```python
from build123d import *

# Parameters (mm, degrees)
SKETCH1_W                   = 26.12
SKETCH1_H                   = 24
SKETCH1_R                   = 1.25
BOSS_EXTRUDE1_DEPTH         = 2
SKETCH4_W                   = 26.12
SKETCH4_H                   = 2
BOSS_EXTRUDE4_DEPTH         = 20
FILLET2_R                   = 2.54
FILLET3_R                   = 1
FILLET4_R                   = 1
FILLET5_R                   = 1
BOSS_EXTRUDE5_DEPTH         = 2
BOSS_EXTRUDE6_DEPTH         = 1
FILLET10_R                  = 1
SKETCH15_R                  = 3.5
BOSS_EXTRUDE7_DEPTH         = 8
M3_5X0_6_TAPPED_HOLE1_D     = 2.9
M3_5X0_6_TAPPED_HOLE1_DEPTH = 10
M3_5X0_6_TAPPED_HOLE1_TIP   = 0.871247898
SKETCH19_R                  = 3.500559702
SKETCH19_R_2                = 1.27
BOSS_EXTRUDE8_DEPTH         = 3
CUT_EXTRUDE1_DEPTH          = 3
FILLET11_R                  = 2.54
SKETCH21_R                  = 1.75
CUT_EXTRUDE2_DEPTH          = 3


with BuildPart() as part:
    # Sketch1 → Boss-Extrude1 (new body)
    with BuildSketch(Plane.XY):
        with Locations((-15.65045068, 0.61225)):
            Rectangle(SKETCH1_W, SKETCH1_H)
        with Locations((-7.12045068, -2.85775)):
            Circle(SKETCH1_R, mode=Mode.SUBTRACT)
        with Locations((-24.18045068, 10.09225)):
            Circle(SKETCH1_R, mode=Mode.SUBTRACT)
    extrude(amount=BOSS_EXTRUDE1_DEPTH)

    # Sketch4 → Boss-Extrude4 (add)
    with BuildSketch(Plane(origin=(0, 0, 0), x_dir=(-1, 0, 0), z_dir=(0, 0, -1))):
        with Locations((15.65045068, -10.38775)):
            Rectangle(SKETCH4_W, SKETCH4_H)
    extrude(amount=BOSS_EXTRUDE4_DEPTH)

    # Fillet2
    fillet2_edges = [part.edges().sort_by_distance(p)[0] for p in [
        (-28.71045068, 12.61225, 1),
    ]]
    fillet(fillet2_edges, radius=FILLET2_R)

    # Fillet3
    fillet3_edges = [part.edges().sort_by_distance(p)[0] for p in [
        (-2.59045068, 12.61225, 1),
    ]]
    fillet(fillet3_edges, radius=FILLET3_R)

    # Fillet4
    fillet4_edges = [part.edges().sort_by_distance(p)[0] for p in [
        (-28.71045068, -10.38775, -20),
        (-2.59045068, -10.38775, -20),
    ]]
    fillet(fillet4_edges, radius=FILLET4_R)

    # Fillet5
    fillet5_edges = [part.edges().sort_by_distance(p)[0] for p in [
        (-15.65045068, -9.38775, 0),
    ]]
    fillet(fillet5_edges, radius=FILLET5_R)

    # Sketch7 → Boss-Extrude5 (add)
    with BuildSketch(Plane.XY.offset(2)):
        with BuildLine():
            Line((-26.610166349, 12.61225), (-21.750735012, 12.61225))
            ThreePointArc((-21.750735012, 12.61225), (-24.18045068, 13.592809702), (-26.610166349, 12.61225))
        make_face()
    extrude(amount=-BOSS_EXTRUDE5_DEPTH)

    # Sketch14 → Boss-Extrude6 (add, symmetric)
    with BuildSketch(Plane.ZY.offset(15.65045068)):
        Polygon((0, 11.61225), (-19, -9.38775), (0, -9.38775), (0, 11.544281389), align=None)
    extrude(amount=BOSS_EXTRUDE6_DEPTH, both=True)

    # Fillet10
    fillet10_edges = [part.edges().sort_by_distance(p)[0] for p in [
        (-14.65045068, -9.094856781, -0.292893219),
        (-16.65045068, -9.094856781, -0.292893219),
        (-14.65045068, 1.61225, 0),
        (-16.65045068, 1.61225, 0),
        (-16.65045068, -9.38775, -10),
        (-14.65045068, -9.38775, -10),
    ]]
    fillet(fillet10_edges, radius=FILLET10_R)

    # Sketch15 → Boss-Extrude7 (add)
    with BuildSketch(Plane.XZ.offset(11.38775)):
        with Locations((-15.65045068, -9)):
            Circle(SKETCH15_R)
    extrude(amount=-BOSS_EXTRUDE7_DEPTH)

    # M3.5x0.6 Tapped Hole1
    with Locations(Plane(origin=(0, -11.38775, 0), x_dir=(-1, 0, 0), z_dir=(0, -1, 0))):
        with Locations((15.65045068, 9)):
            Hole(M3_5X0_6_TAPPED_HOLE1_D / 2, depth=M3_5X0_6_TAPPED_HOLE1_DEPTH)
            with Locations((0, 0, -(M3_5X0_6_TAPPED_HOLE1_DEPTH + M3_5X0_6_TAPPED_HOLE1_TIP / 2))):  # 118° drill point
                Cone(0, M3_5X0_6_TAPPED_HOLE1_D / 2, M3_5X0_6_TAPPED_HOLE1_TIP, mode=Mode.SUBTRACT)

    # Sketch19 → Boss-Extrude8 (add)
    with BuildSketch(Plane(origin=(0, 0, 0), x_dir=(-1, 0, 0), z_dir=(0, 0, -1))):
        with Locations((7.12045068, -2.85775)):
            Circle(SKETCH19_R)
        with Locations((7.12045068, -2.85775)):
            Circle(SKETCH19_R_2, mode=Mode.SUBTRACT)
        with Locations((24.18045068, 10.09225)):
            Circle(SKETCH19_R)
        with Locations((24.18045068, 10.09225)):
            Circle(SKETCH19_R_2, mode=Mode.SUBTRACT)
    extrude(amount=BOSS_EXTRUDE8_DEPTH)

    # Sketch20 → Cut-Extrude1 (cut, through all)
    with BuildSketch(Plane(origin=(0, 0, 0), x_dir=(-1, 0, 0), z_dir=(0, 0, -1))):
        with BuildLine():
            Line((21.027116218, 11.61225), (2.59045068, 11.61225))
            Line((2.59045068, 11.61225), (2.59045068, 12.61225))
            Line((2.59045068, 12.61225), (21.750735012, 12.61225))
            ThreePointArc((21.750735012, 12.61225), (21.344500718, 12.144396691), (21.027116218, 11.61225))
        make_face()
    extrude(amount=-CUT_EXTRUDE1_DEPTH, mode=Mode.SUBTRACT)

    # Fillet11
    fillet11_edges = [part.edges().sort_by_distance(p)[0] for p in [
        (-2.59045068, 11.61225, 1),
    ]]
    fillet(fillet11_edges, radius=FILLET11_R)

    # Sketch21 → Cut-Extrude2 (cut, through all)
    with BuildSketch(Plane(origin=(0, -9.38775, 0), x_dir=(1, 0, 0), z_dir=(0, 1, 0))):
        with Locations((-23.63045068, 14.92)):
            Circle(SKETCH21_R)
        with Locations((-7.67045068, 14.92)):
            Circle(SKETCH21_R)
    extrude(amount=-CUT_EXTRUDE2_DEPTH, mode=Mode.SUBTRACT)


solid = part.part
```
Work out the finished part from the listing and answer in its coordinate system (mm). A direction names the side the tool comes from. Give positions to 0.01 mm unless a question says otherwise; leave off trailing zeros. Loops run counter-clockwise (first coordinate to the right, second up) from the corner with the lowest first, then second, coordinate; pieces in that order, holes last. Notation, with made-up numbers: (84.25, -36) - (90.25, -36) arc R11 cw to (90.25, -28) - close; hole circle Ø11 at (62.25, 33). An arc over 180 degrees is marked (long way). Use CSV: the item, a comma, the result in double quotes. Start each with the question number.
(1) Find the intervals of material crossed by L1, parallel to X at y = -10.2, z = -14.92; L2, parallel to X at y = 10.25, z = -0.5; L3, parallel to Y at x = -25.75, z = -11.75, in increasing order.
(2) Find section A-A, the plane x = -24. Count the separate pieces of the cut face and the enclosed holes in it, plus the area to 3 significant figures.
(3) Find section D-D, the plane z = -14.92. Determine the outline of the cut face in (x, y).
(4) Determine the mould class of faces 1 (the face through (-16.94, -9.09, -3.53)), 2 (the face through (-13, 11.612, 1)), 3 (the face through (-28.425, -10.374, -19.699)) for opening direction Z: released by +Z, released by -Z, zero draft, split by the parting line, or undercut.
(5) A tool of negligible diameter and unlimited length cuts with its end or side. For faces 4 (the face through (-16.94, -9.09, -15.39)), 5 (the face through (-14.365, -9.087, -3.528)), 6 (the face through (-7.1, -4.4, -3)), from which of +Z, -Z, +X, -X, +Y, -Y can it reach the whole face along a straight path? Write none if from no direction.
(6) Find section C-C, the plane y = -4.75. Determine the outline of the cut face in (x, z), plus the area to 3 significant figures.
(7) Each of these flat-tipped pins is pushed along its axis until it touches: pin 1 (0.8 mm diameter, centred on x = -23.5, y = 9.5, fed in from -Z); pin 2 (10 mm diameter, centred on x = -11.5, y = -2.5, fed in from -Z); pin 3 (3 mm diameter, centred on x = -23.63, z = -14.92, fed in from +Y); pin 4 (5 mm diameter, centred on x = -16, z = -8.5, fed in from +Y). Where does it stop, or does it pass through?
(8) Find section B-B, the plane x = -11.5. Determine the outline of the cut face in (y, z), plus the area to 3 significant figures.
Results found:
1,L1,"-28.71 to -25.38, -21.88 to -9.42, -5.92 to -2.59"
1,L2,"-27.68 to -25.44, -22.92 to -20.68, -16.78 to -14.52"
1,L3,"-11.39 to -9.39"
2,separate pieces,"3"
2,enclosed holes,"0"
2,area,"91.8 mm^2"
3,outline,"(-28.71, -11.39) - (-25.38, -11.39) - (-25.38, -9.39) - (-28.71, -9.39) - close; (-21.88, -11.39) - (-9.42, -11.39) - (-9.42, -9.39) - (-13.65, -9.39) arc R1 cw to (-14.65, -8.39) - (-14.65, -4.88) - (-16.65, -4.88) - (-16.65, -8.39) arc R1 cw to (-17.65, -9.39) - (-21.88, -9.39) - close; (-5.92, -11.39) - (-2.59, -11.39) - (-2.59, -9.39) - (-5.92, -9.39) - close"
4,face 1,"undercut"
4,face 2,"zero draft"
4,face 3,"released by -Z"
5,face 4,"-Z, -X, +Y"
5,face 5,"+X, +Y"
5,face 6,"-Z, +X, +Y"
6,outline,"(-28.71, 0) - (-17.65, 0) arc R1 cw to (-16.65, -1) - (-16.65, -5.65) arc R3.5 ccw to (-16.65, -12.35) - (-16.65, -14.8) - (-14.65, -14.8) - (-14.65, -12.35) arc R3.5 ccw to (-14.65, -5.65) - (-14.65, -1) arc R1 cw to (-13.65, 0) - (-10.07, 0) - (-10.07, -3) - (-4.18, -3) - (-4.18, 0) - (-2.59, 0) - (-2.59, 2) - (-28.71, 2) - close; hole circle Ø2.9 at (-15.65, -9)"
6,area,"118 mm^2"
7,pin 1,"z = -3"
7,pin 2,"z = -16.28"
7,pin 3,"through"
7,pin 4,"y = 4.98"
8,outline,"(-11.39, -20) - (-9.39, -20) - (-9.39, -1) arc R1 cw to (-8.39, 0) - (11.61, 0) - (11.61, 2) - (-11.39, 2) - close"
8,area,"86.2 mm^2"
